```python
from build123d import *

# Parameters (mm, degrees)
BOSS_EXTRUDE1_DEPTH = 8
SKETCH2_W           = 1.9
SKETCH2_H           = 2.4
BOSS_EXTRUDE2_DEPTH = 4
SKETCH3_W           = 18
SKETCH3_H           = 2
CUT_EXTRUDE1_DEPTH  = 10
SKETCH4_W           = 9.5
SKETCH4_H           = 20
CUT_EXTRUDE2_DEPTH  = 4
SKETCH5_W           = 9.5
SKETCH5_H           = 20
CUT_EXTRUDE3_DEPTH  = 4


with BuildPart() as part:
    # Sketch1 → Boss-Extrude1 (new body)
    with BuildSketch(Plane(origin=(0, 0, 0), x_dir=(1, 0, 0), z_dir=(0, 1, 0))):
        with BuildLine():
            Line((-18, -10), (-18, -3.5))
            Line((-18, -3.5), (-28, -3.5))
            Line((-28, -3.5), (-28, 3.5))
            Line((-28, 3.5), (-18, 3.5))
            Line((-18, 3.5), (-18, 10))
            ThreePointArc((-18, 10), (-15.656854249, 15.656854249), (-10, 18))
            Line((-10, 18), (10, 18))
            ThreePointArc((10, 18), (15.656854249, 15.656854249), (18, 10))
            Line((18, 10), (18, 9))
            Line((18, 9), (28, 9))
            Line((28, 9), (28, 5))
            Line((28, 5), (18, 5))
            Line((18, 5), (18, -5))
            Line((18, -5), (28, -5))
            Line((28, -5), (28, -9))
            Line((28, -9), (18, -9))
            Line((18, -9), (18, -10))
            ThreePointArc((18, -10), (15.656854249, -15.656854249), (10, -18))
            Line((10, -18), (-10, -18))
            ThreePointArc((-10, -18), (-15.656854249, -15.656854249), (-18, -10))
        make_face()
        with BuildLine():
            Line((-10, -15), (10, -15))
            ThreePointArc((10, -15), (13.535533906, -13.535533906), (15, -10))
            ThreePointArc((15, -10), (12.658876757, -4.136567081), (6.923127464, -1.498028909))
            ThreePointArc((6.923127464, -1.498028909), (5.5, 0), (6.923127464, 1.498028909))
            ThreePointArc((6.923127464, 1.498028909), (12.658876757, 4.136567081), (15, 10))
            ThreePointArc((15, 10), (13.535533906, 13.535533906), (10, 15))
            Line((10, 15), (-10, 15))
            ThreePointArc((-10, 15), (-13.535533906, 13.535533906), (-15, 10))
            ThreePointArc((-15, 10), (-12.658876757, 4.136567081), (-6.923127464, 1.498028909))
            ThreePointArc((-6.923127464, 1.498028909), (-5.5, 0), (-6.923127464, -1.498028909))
            ThreePointArc((-6.923127464, -1.498028909), (-12.658876757, -4.136567081), (-15, -10))
            ThreePointArc((-15, -10), (-13.535533906, -13.535533906), (-10, -15))
        make_face(mode=Mode.SUBTRACT)
    extrude(amount=BOSS_EXTRUDE1_DEPTH)

    # Sketch2 → Boss-Extrude2 (add)
    with BuildSketch(Plane.ZY.offset(28)):
        with Locations((2.55, 6.8)):
            Rectangle(SKETCH2_W, SKETCH2_H)
        with Locations((-2.55, 5.2)):
            Rectangle(SKETCH2_W, SKETCH2_H)
    extrude(amount=BOSS_EXTRUDE2_DEPTH)

    # Sketch3 → Cut-Extrude1 (cut)
    with BuildSketch(Plane(origin=(28, 0, 0), x_dir=(0, 0, -1), z_dir=(1, 0, 0))):
        with Locations((0, 1)):
            Rectangle(SKETCH3_W, SKETCH3_H)
        with Locations((0, 7)):
            Rectangle(SKETCH3_W, SKETCH3_H)
    extrude(amount=-CUT_EXTRUDE1_DEPTH, mode=Mode.SUBTRACT)

    # Sketch4 → Cut-Extrude2 (cut)
    with BuildSketch(Plane.XZ):
        with Locations((10.25, 0)):
            Rectangle(SKETCH4_W, SKETCH4_H)
    extrude(amount=-CUT_EXTRUDE2_DEPTH, mode=Mode.SUBTRACT)

    # Sketch5 → Cut-Extrude3 (cut)
    with BuildSketch(Plane(origin=(0, 8, 0), x_dir=(1, 0, 0), z_dir=(0, 1, 0))):
        with Locations((-10.25, 0)):
            Rectangle(SKETCH5_W, SKETCH5_H)
    extrude(amount=-CUT_EXTRUDE3_DEPTH, mode=Mode.SUBTRACT)


solid = part.part
```
Model file for the job. Use its own axes, mm. A direction names the side the tool comes from. Coordinates: 2 decimals unless noted, no trailing zeros. Order: outer loops, then holes, each group sorted by start corner. A loop starts at its lowest first (then second) coordinate and runs counter-clockwise, first axis right, second up. Notation, with made-up numbers: (31, 80.5) - (84, 80.5) arc R17 cw to (84, 99.5) - close; hole circle Ø9 at (31, 43.25). An arc over 180 degrees is marked (long way). Return JSON: item names as keys, results as strings. Group by question number.
1) Saw through at B-B, the plane x = 22.5. Write the cut outline in (y, z).
2) Saw through at A-A, the plane z = 0. Write the cut outline in (x, y).
3) Probe line 1 (Z direction, x = 5, y = 4.75); line 2 (Z direction, x = 20.5, y = 2.5); line 3 (X direction, y = 4.5, z = 0). List the from-to ranges inside material, lowest first. Write a range as from..to.
4) Flat gauge pins, fed straight in: P1, Ø1.5, axis at x = 19, y = 4.5, coming from the -Z side; P2, Ø4.5, axis at x = 23, y = 3.5, coming from the +Z side; P3, Ø4, axis at x = -26, y = 2, coming from the +Z side. Where does each tip first touch, or does it go through?
5) Saw through at D-D, the plane x = 3. Write the cut outline in (y, z), plus the area to 3 significant figures.
6) Tool access for faces 1 (the flat face through (23, 4, -5)), 2 (the flat face through (-15, 6, 0)), 3 (the cylindrical face through (-5.5, 2, 0)): list every direction of +Z, -Z, +X, -X, +Y, -Y with a clear straight run to the whole face (end or side of a thin tool).
7) Mould opens along Z. For faces 4 (the flat face through (23, 4, 9)), 5 (the flat face through (-30, 5.6, 3)), 6 (the flat face through (-30, 7, 1.6)) say: released by +Z, released by -Z, zero draft, split by the parting line, or undercut.
Values found:
{
 "1": {"outline": "(2, -9) - (6, -9) - (6, -5) - (2, -5) - close; (2, 5) - (6, 5) - (6, 9) - (2, 9) - close"},
 "2": {"outline": "(-28, 0) - (-5.5, 0) - (-5.5, 4) - (-15, 4) - (-15, 8) - (-28, 8) - close; (5.5, 4) - (15, 4) - (15, 0) - (18, 0) - (18, 8) - (5.5, 8) - close"},
 "3": {"line 1": "z = -18..-15, 15..18", "line 2": "z = -9..-5, 5..9", "line 3": "x = -28..-15, 5.5..18"},
 "4": {"P1": "stops at z = -9", "P2": "stops at z = 9", "P3": "stops at z = 3.5"},
 "5": {"outline": "(0, -18) - (8, -18) - (8, -15) - (0, -15) - close; (0, 15) - (8, 15) - (8, 18) - (0, 18) - close", "area": "48.0 mm²"},
 "6": {"face 1": "+X, +Y, -Y", "face 2": "+Y", "face 3": "+Y, -Y"},
 "7": {"face 4": "released by +Z", "face 5": "zero draft", "face 6": "undercut"}
}
